```python
from build123d import *

# Parameters (mm, degrees)
SKETCH2_W           = 140
SKETCH2_H           = 140
SKETCH2_R           = 1.6
SKETCH2_R_2         = 1.4
BOSS_EXTRUDE2_DEPTH = 3
SKETCH3_W           = 14
SKETCH3_H           = 3
SKETCH3_W_2         = 3
SKETCH3_H_2         = 14
CUT_EXTRUDE1_DEPTH  = 10


with BuildPart() as part:
    # Sketch2 → Boss-Extrude2 (new body)
    with BuildSketch(Plane(origin=(0, 0, 0), x_dir=(1, 0, 0), z_dir=(0, 1, 0))):
        Rectangle(SKETCH2_W, SKETCH2_H)
        with Locations((-17.011581703, 44.949159058)):
            Circle(SKETCH2_R, mode=Mode.SUBTRACT)
        with Locations((-18.611581703, -3.350840942)):
            Circle(SKETCH2_R, mode=Mode.SUBTRACT)
        with Locations((33.788418297, 29.649159058)):
            Circle(SKETCH2_R, mode=Mode.SUBTRACT)
        with Locations((33.788418297, 1.749159058)):
            Circle(SKETCH2_R, mode=Mode.SUBTRACT)
        with Locations((0, 60)):
            Circle(SKETCH2_R, mode=Mode.SUBTRACT)
        with Locations((-60, 0)):
            Circle(SKETCH2_R, mode=Mode.SUBTRACT)
        with Locations((0, -60)):
            Circle(SKETCH2_R, mode=Mode.SUBTRACT)
        with Locations((60, 0)):
            Circle(SKETCH2_R, mode=Mode.SUBTRACT)
        with Locations((-45, 60)):
            Circle(SKETCH2_R, mode=Mode.SUBTRACT)
        with Locations((45, 60)):
            Circle(SKETCH2_R, mode=Mode.SUBTRACT)
        with Locations((-45, -60)):
            Circle(SKETCH2_R, mode=Mode.SUBTRACT)
        with Locations((45, -60)):
            Circle(SKETCH2_R, mode=Mode.SUBTRACT)
        with Locations((-0.030225379, -18.62367845)):
            Circle(SKETCH2_R_2, mode=Mode.SUBTRACT)
        with Locations((-13.780225379, -40.12367845)):
            Circle(SKETCH2_R_2, mode=Mode.SUBTRACT)
        with Locations((13.719774621, -40.12367845)):
            Circle(SKETCH2_R_2, mode=Mode.SUBTRACT)
    extrude(amount=BOSS_EXTRUDE2_DEPTH)

    # Sketch3 → Cut-Extrude1 (cut)
    with BuildSketch(Plane(origin=(0, 3, 0), x_dir=(1, 0, 0), z_dir=(0, 1, 0))):
        with Locations((23, -68.5)):
            Rectangle(SKETCH3_W, SKETCH3_H)
        with Locations((23, 68.5)):
            Rectangle(SKETCH3_W, SKETCH3_H)
        with Locations((-23, 68.5)):
            Rectangle(SKETCH3_W, SKETCH3_H)
        with Locations((-23, -68.5)):
            Rectangle(SKETCH3_W, SKETCH3_H)
        with Locations((68.5, -23)):
            Rectangle(SKETCH3_W_2, SKETCH3_H_2)
        with Locations((68.5, 23)):
            Rectangle(SKETCH3_W_2, SKETCH3_H_2)
        with Locations((-68.5, 23)):
            Rectangle(SKETCH3_W_2, SKETCH3_H_2)
        with Locations((-68.5, -23)):
            Rectangle(SKETCH3_W_2, SKETCH3_H_2)
    extrude(amount=-CUT_EXTRUDE1_DEPTH, mode=Mode.SUBTRACT)


solid = part.part
```
For this review, take the finished solid that the model builds, in its own axes (mm). A direction names the side the tool comes from. Coordinates: 2 decimals unless noted, no trailing zeros. Loops run counter-clockwise (first coordinate to the right, second up) from the corner with the lowest first, then second, coordinate; pieces in that order, holes last. Notation, with made-up numbers: (85, 40) -> (109, 40) arc R12 ccw to (109, 59) -> close; hole circle Ø7 at (-13, 47.5). An arc over 180 degrees is marked (long way). Return JSON: item names as keys, results as strings. Group by question number.
(1) Tool access review of faces 1 (the flat face through (-23, 2, -67)), 2 (the flat face through (-30, 2, 69)), 3 (the flat face through (-69, 2, -30)), 4 (the flat face through (50, 1, 70)): name each direction out of +Z, -Z, +X, -X, +Y, -Y from which nothing blocks a thin tool from reaching the whole face with its end or side.
(2) Consider section B-B, the plane z = 60. Give the boundary of the cut face in (x, y).
(3) For pin 1 Ø1.7 at (x, z) = (-13.78, 40.12) entering from +Y; pin 2 Ø1.5 at (y, z) = (1, 24.5) entering from +X; pin 3 Ø0.9 at (x, y) = (-26.5, 1) entering from -Z, all flat-tipped, find the tip position at first contact; note any pin that passes through.
(4) To check wall thickness, follow L1, parallel to X at y = 0.8, z = 60; L2, parallel to Z at x = 0, y = 0.75; L3, parallel to X at y = 2.05, z = -16.5. State the ranges of each line that lie inside material, in increasing order.
(5) Mouldability with a two-part tool opening along Z and no side actions: class faces 5 (the flat face through (-50, 1, 70)), 6 (the flat face through (-1, 0, -1)), 7 (the flat face through (-69, 2, 30)) as pulls with the +Z half, pulls with the -Z half, needs draft (parallel to the pull), parting line crosses it, or undercut.
(6) Consider section A-A, the plane x = -60. Give the boundary of the cut face in (y, z).
(7) Consider section D-D, the plane z = -18. Give the boundary of the cut face in (x, y), plus the area to 3 significant figures.
(8) Consider section C-C, the plane x = -45. Give the boundary of the cut face in (y, z).
Results below:
{
 "1": {"face 1": "-Z, +Y, -Y", "face 2": "+Z, +Y, -Y", "face 3": "-X, +Y, -Y", "face 4": "+Z, +X, -X, +Y, -Y"},
 "2": {"outline": "(-70, 0) -> (-46.6, 0) -> (-46.6, 3) -> (-70, 3) -> close; (-43.4, 0) -> (-1.6, 0) -> (-1.6, 3) -> (-43.4, 3) -> close; (1.6, 0) -> (43.4, 0) -> (43.4, 3) -> (1.6, 3) -> close; (46.6, 0) -> (70, 0) -> (70, 3) -> (46.6, 3) -> close"},
 "3": {"pin 1": "passes through", "pin 2": "stops at x = 67", "pin 3": "stops at z = -67"},
 "4": {"L1": "x = -70 to -46.6, -43.4 to -1.6, 1.6 to 43.4, 46.6 to 70", "L2": "z = -70 to -61.6, -58.4 to 17.22, 20.02 to 58.4, 61.6 to 70", "L3": "x = -67 to 67"},
 "5": {"face 5": "pulls with the +Z half", "face 6": "needs draft", "face 7": "undercut"},
 "6": {"outline": "(0, -70) -> (3, -70) -> (3, -1.6) -> (0, -1.6) -> close; (0, 1.6) -> (3, 1.6) -> (3, 70) -> (0, 70) -> close"},
 "7": {"outline": "(-67, 0) -> (67, 0) -> (67, 3) -> (-67, 3) -> close", "area": "402 mm2"},
 "8": {"outline": "(0, -70) -> (3, -70) -> (3, -61.6) -> (0, -61.6) -> close; (0, -58.4) -> (3, -58.4) -> (3, 58.4) -> (0, 58.4) -> close; (0, 61.6) -> (3, 61.6) -> (3, 70) -> (0, 70) -> close"}
}
